Model file for the job. Use its own axes, mm. A direction names the side the tool comes from. Coordinates: 2 decimals unless noted, no trailing zeros. Loops run counter-clockwise (first coordinate to the right, second up) from the corner with the lowest first, then second, coordinate; pieces in that order, holes last. Notation, with made-up numbers: (74.5, 50) -> (103.5, 50) arc R34 ccw to (103.5, 88) -> close; hole circle Ø11 at (-37.5, 54). An arc over 180 degrees is marked (long way). Use one line per item in the form item = value.
```python
from build123d import *

# Parameters (mm, degrees)
F0_R     = 63.5
F0_R_2   = 1.5875
F1_DEPTH = 38.1


with BuildPart() as f1:
    # F0 (on Front) → F1 (new body)
    with BuildSketch(Plane.XZ):
        with Locations((-16.125669, 21.278876)):
            Circle(F0_R)
        with BuildLine():
            ThreePointArc((-19.895006, -34.47385), (-55.147708, -18.71931), (-71.768271, 16.133457))
            Line((-71.768271, 16.133457), (-19.895006, 16.133457))
            Line((-19.895006, 16.133457), (-19.895006, -34.47385))
        make_face(mode=Mode.SUBTRACT)
        with BuildLine():
            Line((-11.770886, -34.431179), (-11.770886, 16.133457))
            Line((-11.770886, 16.133457), (39.516932, 16.133457))
            ThreePointArc((39.516932, 16.133457), (23.105914, -18.513802), (-11.770886, -34.431179))
        make_face(mode=Mode.SUBTRACT)
        with BuildLine():
            ThreePointArc((-71.796996, 26.103588), (-55.262784, 61.16447), (-19.895006, 77.031602))
            Line((-19.895006, 77.031602), (-19.895006, 26.103588))
            Line((-19.895006, 26.103588), (-71.796996, 26.103588))
        make_face(mode=Mode.SUBTRACT)
        with Locations((-16.125669, 21.278876)):
            Circle(F0_R_2, mode=Mode.SUBTRACT)
        with BuildLine():
            Line((-11.770886, 26.103588), (-11.770886, 76.988931))
            ThreePointArc((-11.770886, 76.988931), (23.220398, 60.958359), (39.545657, 26.103588))
            Line((39.545657, 26.103588), (-11.770886, 26.103588))
        make_face(mode=Mode.SUBTRACT)
    extrude(amount=F1_DEPTH)


solid = f1.part
```
Q1. Which spindle directions (+Z, -Z, +X, -X, +Y, -Y) get a long thin tool onto all of the face, cutting with end or side? Do faces 4 (the face through (-17, 0, 8)), 5 (the face through (-45, -19, 26.104)). Say none if no direction does.
Result:
face_4 = +Z, -Z, +X, -X, +Y
face_5 = +Y, -Y
Q2. Mould opens along X. For faces 1 (the face through (-11.771, -19, 51)), 2 (the face through (18.012, -18.783, 74.822)), 3 (the face through (-17, -38.1, 8)) say: released by +X, released by -X, zero draft, split by the parting line, or undercut.
Result:
face_1 = undercut
face_2 = split by the parting line
face_3 = zero draft
Q3. Pin check, flat tips, straight feed: pin 1 Ø6 at (x, y) = (5.5, -4.5) entering from -Z; pin 2 Ø19 at (x, y) = (-42.5, -16.5) entering from +Z; pin 3 Ø2 at (y, z) = (-23, -29.5) entering from +X; pin 4 Ø6 at (x, z) = (6.5, 30.5) entering from -Y. Stop position of each tip, or through.
Result:
pin_1 = -39.43
pin_2 = 82.5
pin_3 = 23.3
pin_4 = through
Q4. Band-saw the part on A-A, the plane z = 38.5. Write the cut outline in (x, y) (3 decimals), and give its area (3 significant figures).
Result:
outline = (-77.246, -38.1) -> (-69.286, -38.1) -> (-69.286, 0) -> (-77.246, 0) -> close; (-19.895, -38.1) -> (-11.771, -38.1) -> (-11.771, 0) -> (-19.895, 0) -> close; (37.035, -38.1) -> (44.995, -38.1) -> (44.995, 0) -> (37.035, 0) -> close
area = 916 mm2
Q5. Wall check: line 1 along X through (y, z) = (-35, 42) (3 decimals); line 2 along X through (y, z) = (-34.5, 72) (1 decimal); line 3 along Z through (x, y) = (-66.5, -26.5). Give the ranges that are in metal, low to high.
Result:
line_1 = -76.15 to -68.022, -19.895 to -11.771, 35.77 to 43.898
line_2 = -54.3 to -39.6, -19.9 to -11.8, 7.3 to 22.1
line_3 = -17.38 to -2.91, 16.13 to 26.1, 45.47 to 59.94
Q6. Band-saw the part on C-C, the plane y = -3.5. Write the cut outline in (x, z) (1 decimal), and give its area (3 significant figures).
Result:
outline = circle Ø127 at (-16.1, 21.3); hole (-71.8, 16.1) arc R55.9 ccw to (-19.9, -34.5) -> (-19.9, 16.1) -> close; hole (-71.8, 26.1) -> (-19.9, 26.1) -> (-19.9, 77) arc R55.9 ccw to start; hole circle Ø3.2 at (-16.1, 21.3); hole (-11.8, -34.4) arc R55.9 ccw to (39.5, 16.1) -> (-11.8, 16.1) -> close; hole (-11.8, 26.1) -> (39.5, 26.1) arc R55.9 ccw to (-11.8, 77) -> close
area = 4,790 mm2
Q7. Band-saw the part on B-B, the plane x = -46.5. Write the cut outline in (y, z) (3 decimals), and give its area (3 significant figures).
Result:
outline = (-38.1, -34.485) -> (0, -34.485) -> (0, -25.625) -> (-38.1, -25.625) -> close; (-38.1, 16.133) -> (0, 16.133) -> (0, 26.104) -> (-38.1, 26.104) -> close; (-38.1, 68.183) -> (0, 68.183) -> (0, 77.043) -> (-38.1, 77.043) -> close
area = 1,060 mm2
